from build123d import *

# Parameters (mm, degrees)
SKETCH1_W           = 50
SKETCH1_H           = 25
BOSS_EXTRUDE1_DEPTH = 10
SKETCH2_R           = 1.8
CUT_EXTRUDE1_DEPTH  = 57.789083458
SKETCH3_W           = 4
SKETCH3_H           = 15
CUT_EXTRUDE2_DEPTH  = 10
SKETCH6_W           = 14.8
SKETCH6_H           = 15
CUT_EXTRUDE3_DEPTH  = 57.789083458


with BuildPart() as part:
    # Sketch1 → Boss-Extrude1 (new body)
    with BuildSketch(Plane.XY):
        with Locations((25, 12.5)):
            Rectangle(SKETCH1_W, SKETCH1_H)
    extrude(amount=BOSS_EXTRUDE1_DEPTH)

    # Sketch2 → Cut-Extrude1 (cut, through all)
    with BuildSketch(Plane(origin=(0, 25, 0), x_dir=(1, 0, 0), z_dir=(0, 1, 0))):
        with Locations(Location((10, -5, 0), (0, 0, 180))):
            Circle(SKETCH2_R)
        with Locations(Location((40, -5, 0), (0, 0, 180))):
            Circle(SKETCH2_R)
    extrude(amount=-CUT_EXTRUDE1_DEPTH, mode=Mode.SUBTRACT)

    # Sketch3 → Cut-Extrude2 (cut)
    with BuildSketch(Plane.XY.offset(10)):
        with Locations((25, 17.5)):
            Rectangle(SKETCH3_W, SKETCH3_H)
    extrude(amount=-CUT_EXTRUDE2_DEPTH, mode=Mode.SUBTRACT)

    # Sketch6 → Cut-Extrude3 (cut, through all)
    with BuildSketch(Plane.XY.offset(10)):
        with Locations((7.4, 7.5)):
            Rectangle(SKETCH6_W, SKETCH6_H)
        with Locations((42.6, 7.5)):
            Rectangle(SKETCH6_W, SKETCH6_H)
    extrude(amount=-CUT_EXTRUDE3_DEPTH, mode=Mode.SUBTRACT)


solid = part.part
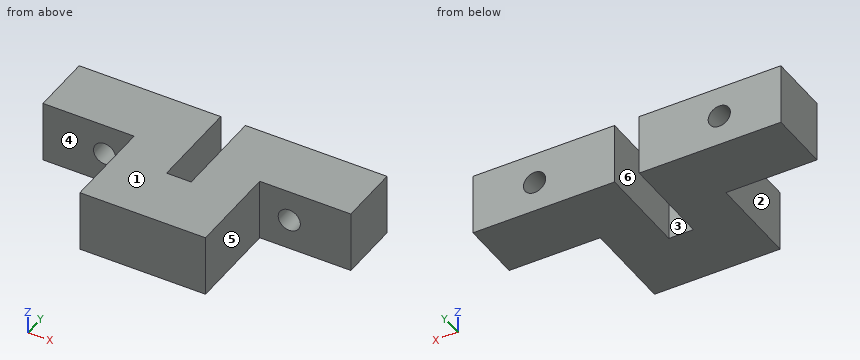
Geometry check sheet. Reference: the model listing, model coordinates, mm. Face numbers are marked on the shaded views. A direction names the side the tool comes from. Round coordinates to 2 decimals unless told otherwise and drop trailing zeros. Order: outer loops, then holes, each group sorted by start corner. A loop starts at its lowest first (then second) coordinate and runs counter-clockwise, first axis right, second up. Notation, with made-up numbers: (7, 7.5) - (39, 7.5) arc R16 cw to (39, 24.5) - close; hole circle Ø10 at (16, 87). An arc over 180 degrees is marked (long way). One line per question, with ' | ' between items. Start each with the question number.
(1) Sectioned sample at B-B on y = 18.5. Record the cut outline in (x, z).
(2) Sectioned sample at C-C on x = 40. Record the cut outline in (y, z).
(3) Depth check by flat-ended pin: pin 1 Ø5 at (y, z) = (7.5, 7) entering from +X; pin 2 Ø5 at (x, z) = (39.5, 4) entering from -Y; pin 3 Ø3 at (y, z) = (11, 7.5) entering from -X. Enter the tip coordinate at first touch or a pass-through.
(4) Thickness scan on L1, parallel to X at y = 12.25, z = 7.5; L2, parallel to X at y = 17.5, z = 4.75; L3, parallel to X at y = 17, z = 0.5. Record the ranges inside material, lowest first. Write a range as [from, to].
(5) Release check for a two-part mould opening along X. For the marked faces 1, 2 and 3 record: released by +X, released by -X, zero draft, split by the parting line, or undercut.
(6) Access from +Z, -Z, +X, -X, +Y, -Y to the whole of each face (thin tool, end or side, straight path). Record for the marked faces 4, 5 and 6.
(7) Sectioned sample at D-D on z = 8. Record the cut outline in (x, y), and give its area (3 significant figures).
(8) Sectioned sample at A-A on z = 5. Record the cut outline in (x, y), and give its area (3 significant figures).
Conclusion:
1) outline: (0, 0) - (23, 0) - (23, 10) - (0, 10) - close; (27, 0) - (50, 0) - (50, 10) - (27, 10) - close; hole circle Ø3.6 at (10, 5); hole circle Ø3.6 at (40, 5)
2) outline: (15, 0) - (25, 0) - (25, 3.2) - (15, 3.2) - close; (15, 6.8) - (25, 6.8) - (25, 10) - (15, 10) - close
3) pin 1: stops at x = 35.2 | pin 2: stops at y = 15 | pin 3: stops at x = 14.8
4) L1: x = [14.8, 23], [27, 35.2] | L2: x = [0, 8.22], [11.78, 23], [27, 38.22], [41.78, 50] | L3: x = [0, 23], [27, 50]
5) face 1: zero draft | face 2: released by -X | face 3: undercut
6) face 4: +Z, -Z, -X, -Y | face 5: +Z, -Z, +X, -Y | face 6: +Z, -Z, +Y
7) outline: (0, 15) - (14.8, 15) - (14.8, 0) - (35.2, 0) - (35.2, 15) - (50, 15) - (50, 25) - (27, 25) - (27, 10) - (23, 10) - (23, 25) - (0, 25) - close | area: 746 mm2
8) outline: (0, 15) - (8.2, 15) - (8.2, 25) - (0, 25) - close; (11.8, 15) - (14.8, 15) - (14.8, 0) - (35.2, 0) - (35.2, 15) - (38.2, 15) - (38.2, 25) - (27, 25) - (27, 10) - (23, 10) - (23, 25) - (11.8, 25) - close; (41.8, 15) - (50, 15) - (50, 25) - (41.8, 25) - close | area: 674 mm2
